```python
from build123d import *

# Parameters (mm, degrees)
SKIZZE1_W                                 = 230
SKIZZE1_H                                 = 230
AUFSATZ_LINEAR_AUSTRAGEN1_DEPTH           = 15
F_15_0_15_DURCHMESSER_BOHRUNG1_D          = 15
F_3_4_3_4_DURCHMESSER_BOHRUNG1_AT_2_COUNT = 2
F_3_4_3_4_DURCHMESSER_BOHRUNG1_AT_2_PITCH = 26
F_3_4_3_4_DURCHMESSER_BOHRUNG1_AT_3_COUNT = 2
F_3_4_3_4_DURCHMESSER_BOHRUNG1_AT_3_PITCH = 26
F_3_4_3_4_DURCHMESSER_BOHRUNG1_AT_4_COUNT = 2
F_3_4_3_4_DURCHMESSER_BOHRUNG1_AT_4_PITCH = 36.769552622
F_22_5_22_5_DURCHMESSER_BOHRUNG1_D        = 22.5
F_7_0_7_DURCHMESSER_BOHRUNG1_D            = 7
VERRUNDUNG5_R                             = 15
VERRUNDUNG6_R                             = 2
M8_GEWINDEBOHRUNG1_D                      = 6.8
M8_GEWINDEBOHRUNG1_DEPTH                  = 30
M8_GEWINDEBOHRUNG1_TIP                    = 2.042926105


with BuildPart() as part:
    # Skizze1 → Aufsatz-Linear austragen1 (new body)
    with BuildSketch(Plane(origin=(0, 0, 0), x_dir=(1, 0, 0), z_dir=(0, 1, 0))):
        Rectangle(SKIZZE1_W, SKIZZE1_H)
    extrude(amount=AUFSATZ_LINEAR_AUSTRAGEN1_DEPTH)

    # Ø15.0 (15) Durchmesser Bohrung1 (through all)
    with Locations(Plane(origin=(0, 15, 0), x_dir=(1, 0, 0), z_dir=(0, 1, 0))):
        with Locations((-81.223039609, 90), (71.525536654, 90)):
            Hole(F_15_0_15_DURCHMESSER_BOHRUNG1_D / 2)

    # Skizze9 → Ø3.4 (3.4) Durchmesser Bohrung1 (revolve, cut)
    with BuildSketch(Plane(origin=(-13, 15, -103), x_dir=(0, 0, 1), z_dir=(1, 0, 0))):
        Polygon((0, 0), (0, 15), (1.725, 15), (1.7, 14.975), (1.7, 0.025), (1.725, 0), align=None)
    f_3_4_3_4_durchmesser_bohrung1 = revolve(axis=Axis((-13, 21.35, -103), (0, -1, 0)), mode=Mode.SUBTRACT)

    # Ø3.4 (3.4) Durchmesser Bohrung1 at 2: Ø3.4 (3.4) Durchmesser Bohrung1 ×2
    with Locations(*[(i * F_3_4_3_4_DURCHMESSER_BOHRUNG1_AT_2_PITCH, 0, 0) for i in range(1, F_3_4_3_4_DURCHMESSER_BOHRUNG1_AT_2_COUNT)]):
        add(f_3_4_3_4_durchmesser_bohrung1, mode=Mode.SUBTRACT)

    # Ø3.4 (3.4) Durchmesser Bohrung1 at 3: Ø3.4 (3.4) Durchmesser Bohrung1 ×2
    with Locations(*[(0, 0, i * F_3_4_3_4_DURCHMESSER_BOHRUNG1_AT_3_PITCH) for i in range(1, F_3_4_3_4_DURCHMESSER_BOHRUNG1_AT_3_COUNT)]):
        add(f_3_4_3_4_durchmesser_bohrung1, mode=Mode.SUBTRACT)

    # Ø3.4 (3.4) Durchmesser Bohrung1 at 4: Ø3.4 (3.4) Durchmesser Bohrung1 ×2
    with Locations(*[Vector(0.7071067811865476, 0, 0.7071067811865475) * (i * F_3_4_3_4_DURCHMESSER_BOHRUNG1_AT_4_PITCH) for i in range(1, F_3_4_3_4_DURCHMESSER_BOHRUNG1_AT_4_COUNT)]):
        add(f_3_4_3_4_durchmesser_bohrung1, mode=Mode.SUBTRACT)

    # Ø22.5 (22.5) Durchmesser Bohrung1 (through all)
    with Locations(Plane(origin=(0, 15, 0), x_dir=(1, 0, 0), z_dir=(0, 1, 0))):
        with Locations((0, 90)):
            Hole(F_22_5_22_5_DURCHMESSER_BOHRUNG1_D / 2)

    # Ø7.0 (7) Durchmesser Bohrung1 (through all)
    with Locations(Plane(origin=(0, 15, 0), x_dir=(1, 0, 0), z_dir=(0, 1, 0))):
        with Locations((-100, -40), (-100, -100), (100, -40), (100, -100)):
            Hole(F_7_0_7_DURCHMESSER_BOHRUNG1_D / 2)

    # Verrundung5
    verrundung5_edges = [part.edges().sort_by_distance(p)[0] for p in [
        (-115, 7.5, -115),
        (115, 7.5, -115),
    ]]
    fillet(verrundung5_edges, radius=VERRUNDUNG5_R)

    # Verrundung6
    verrundung6_edges = [part.edges().sort_by_distance(p)[0] for p in [
        (115, 7.5, 115),
        (-115, 7.5, 115),
    ]]
    fillet(verrundung6_edges, radius=VERRUNDUNG6_R)

    # M8 Gewindebohrung1
    with Locations(Plane.XY.offset(115)):
        with Locations((-85, 7.5), (85, 7.5)):
            Hole(M8_GEWINDEBOHRUNG1_D / 2, depth=M8_GEWINDEBOHRUNG1_DEPTH)
            with Locations((0, 0, -(M8_GEWINDEBOHRUNG1_DEPTH + M8_GEWINDEBOHRUNG1_TIP / 2))):  # 118° drill point
                Cone(0, M8_GEWINDEBOHRUNG1_D / 2, M8_GEWINDEBOHRUNG1_TIP, mode=Mode.SUBTRACT)


solid = part.part
```
Model file for the job. Use its own axes, mm. A direction names the side the tool comes from. Coordinates: 2 decimals unless noted, no trailing zeros. Loops run counter-clockwise (first coordinate to the right, second up) from the corner with the lowest first, then second, coordinate; pieces in that order, holes last. Notation, with made-up numbers: (66.5, 74.5) - (72.5, 74.5) arc R22 ccw to (72.5, 111.5) - close; hole circle Ø3 at (24.5, 9.5). An arc over 180 degrees is marked (long way). Answer as a JSON object with one key per item and string values. Group by question number.
(1) Cut at A-A (x = 0). Give the cut face in (y, z).
(2) Two-plate mould, pull along Y, no slides. Class faces 3 (the face through (-2, 15, -2)), 4 (the face through (-110.72, 7.6, -110.49)), 5 (the face through (84.41, 7.53, 83.31)): released by +Y, released by -Y, zero draft, split by the parting line, or undercut.
(3) Flat gauge pins, fed straight in: pin 1 (4 mm diameter, centred on x = 100, z = 40, fed in from +Y); pin 2 (4 mm diameter, centred on x = -3, z = -19, fed in from -Y). Where does each tip first touch, or does it go through?
(4) Probe line 1 along Z through (x, y) = (-100, 6); line 2 along Z through (x, y) = (-13, 3.75); line 3 along X through (y, z) = (9.5, 40). List the from-to ranges inside material, lowest first.
(5) Tool access for faces 1 (the face through (87.698, 5.431, 99.79)), 2 (the face through (1.465, 7.395, -101.154)): list every direction of +Z, -Z, +X, -X, +Y, -Y with a clear straight run to the whole face (end or side of a thin tool).
(6) Cut at B-B (z = -90). Give the cut face in (x, y), then the cut area to 3 significant figures.
(7) Cut at C-C (x = 70). Give the cut face in (y, z).
Geometry says:
{
 "1": {"outline": "(0, -115) - (15, -115) - (15, -101.25) - (0, -101.25) - close; (0, -78.75) - (15, -78.75) - (15, 115) - (0, 115) - close"},
 "2": {"face 3": "released by +Y", "face 4": "zero draft", "face 5": "undercut"},
 "3": {"pin 1": "passes through", "pin 2": "stops at y = 0"},
 "4": {"line 1": "z = -115 to 36.5, 43.5 to 96.5, 103.5 to 115", "line 2": "z = -115 to -104.7, -101.3 to -78.7, -75.3 to 115", "line 3": "x = -115 to -103.5, -96.5 to 96.5, 103.5 to 115"},
 "5": {"face 1": "+Z", "face 2": "+Y, -Y"},
 "6": {"outline": "(-115, 0) - (-88.72, 0) - (-88.72, 15) - (-115, 15) - close; (-73.72, 0) - (-11.25, 0) - (-11.25, 15) - (-73.72, 15) - close; (11.25, 0) - (64.03, 0) - (64.03, 15) - (11.25, 15) - close; (79.03, 0) - (115, 0) - (115, 15) - (79.03, 15) - close", "area": "2,660 mm^2"},
 "7": {"outline": "(0, -115) - (15, -115) - (15, -97.34) - (0, -97.34) - close; (0, -82.66) - (15, -82.66) - (15, 115) - (0, 115) - close"}
}
